CAD build for the part. Positions are in the model's coordinates, mm. A direction names the side the tool comes from. Round coordinates to 2 decimals unless told otherwise and drop trailing zeros. Write each loop counter-clockwise with the first axis right and the second up, starting at its lowest first coordinate (ties: lowest second). Pieces come first, ordered by that corner, then holes. Notation, with made-up numbers: (23, 32) -> (60, 32) arc R19 cw to (60, 57) -> close; hole circle Ø4 at (13.25, 81). An arc over 180 degrees is marked (long way). Put each result on its own line as item: value. Start each with the question number.
1. Saw through at C-C on y = 14. List the corners of the cut face in (x, z) (1 decimal).
2. Flat gauge pins, fed straight in: P1, Ø4, axis at x = 4.76, y = 4.76, coming from the -Z side; P2, Ø5, axis at y = 2.5, z = 48, coming from the -X side; P3, Ø1.5, axis at y = 14, z = 32, coming from the +X side (3 decimals). Where does each tip first touch, or does it go through?
3. Drill centre lines: line 1 (Y direction, x = 4.75, z = 38.5); line 2 (Z direction, x = 4.75, y = 15.5); line 3 (Z direction, x = 12.5, y = 4). Where is each one in solid material? Low to high. Write a range as from..to.
4. Pull direction X, two halves, no side cores. Call faces 1 (the cylindrical face through (12.234, 4.829, 5.409)), 2 (the flat face through (9.525, 14, 32)), 3 (the cylindrical face through (4.83, 14.01, 62.46)): pulls with the +X half, pulls with the -X half, needs draft (parallel to the pull), parting line crosses it, or undercut.
5. 3-axis set-ups, long thin cutter, end or side, ignore diameter. For faces 4 (the flat face through (7, 8, 65.088)), 5 (the flat face through (14, 9.525, 32)): which of +Z, -Z, +X, -X, +Y, -Y reach the whole face in a straight line?
6. Saw through at D-D on y = 8. List the corners of the cut face in (x, z).
7. Saw through at A-A on x = 6.25. State how many separate pieces and enclosed holes the cut face has, and give its area (3 significant figures).
from build123d import *

# Parameters (mm, degrees)
F0_R     = 2.15265
F1_DEPTH = 65.0875
F2_R     = 2.15265
F3_DEPTH = 9.525
F4_R     = 2.15265
F5_DEPTH = 9.525


with BuildPart() as f1:
    # F0 (on Top) → F1 (new body)
    with BuildSketch(Plane.XY):
        Polygon((0, 19.05), (0, 0), (19.05, 0), (19.05, 9.525), (9.525, 9.525), (9.525, 19.05), align=None)
        with Locations((4.7625, 4.7625)):
            Circle(F0_R, mode=Mode.SUBTRACT)
    extrude(amount=F1_DEPTH)

    # F2 (on face) → F3 (cut, through all)
    with BuildSketch(Plane.YZ.offset(9.525)):
        with Locations((14.2875, 60.325)):
            Circle(F2_R)
        with Locations((14.2875, 14.2875)):
            Circle(F2_R)
    extrude(amount=-F3_DEPTH, mode=Mode.SUBTRACT)

    # F4 (on face) → F5 (cut, through all)
    with BuildSketch(Plane(origin=(0, 9.525, 0), x_dir=(-1, 0, 0), z_dir=(0, 1, 0))):
        with Locations((-14.2875, 50.8)):
            Circle(F4_R)
        with Locations((-14.2875, 4.7625)):
            Circle(F4_R)
    extrude(amount=-F5_DEPTH, mode=Mode.SUBTRACT)


solid = f1.part
Return value:
1. outline: (0, 0) -> (9.5, 0) -> (9.5, 12.2) -> (0, 12.2) -> close; (0, 16.4) -> (9.5, 16.4) -> (9.5, 58.2) -> (0, 58.2) -> close; (0, 62.5) -> (9.5, 62.5) -> (9.5, 65.1) -> (0, 65.1) -> close
2. P1: passes through
2. P2: stops at x = 0
2. P3: stops at x = 9.525
3. line 1: y = 0..2.61, 6.92..19.05
3. line 2: z = 0..12.51, 16.07..58.55, 62.1..65.09
3. line 3: z = 0..3.56, 5.96..49.6, 52..65.09
4. face 1: undercut
4. face 2: pulls with the +X half
4. face 3: needs draft
5. face 4: +Z, +X, -X, +Y, -Y
5. face 5: +Z, -Z, +X, +Y
6. outline: (0, 0) -> (19.05, 0) -> (19.05, 65.09) -> (0, 65.09) -> close; hole circle Ø4.31 at (14.29, 4.76); hole circle Ø4.31 at (14.29, 50.8)
7. separate pieces: 2
7. enclosed holes: 2
7. area: 1,010 mm^2
